Read the model definition and answer for the solid it produces. Units are mm, in the model's axes. Face numbers are marked on the shaded views. A direction names the side the tool comes from. Coordinates: 2 decimals unless noted, no trailing zeros. Loops run counter-clockwise (first coordinate to the right, second up) from the corner with the lowest first, then second, coordinate; pieces in that order, holes last.
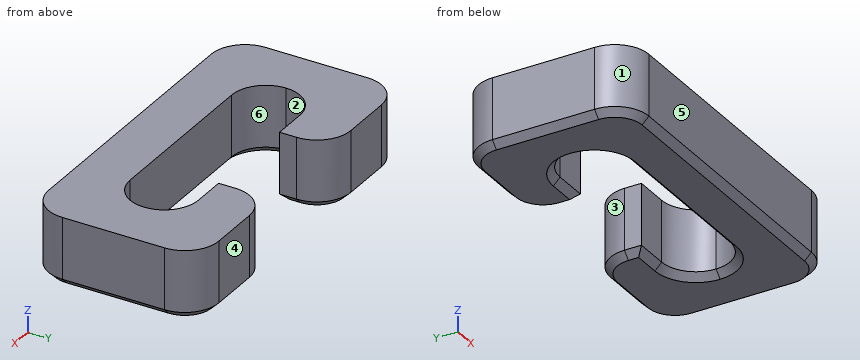
from build123d import *

# Parameters (mm, degrees)
F1_DEPTH = 2
F2_R     = 0.99999
F3_SIZE  = 0.2


# Not quite as in the source:
# - a fillet or chamfer is up to 0.001 mm smaller than in the source, because OpenCascade refuses the exact size


with BuildPart() as f1:
    # F0 (on Top) → F1 (new body)
    with BuildSketch(Plane.XY):
        Polygon((3.5, 0), (0, 0), (-3.5, 0), (-3.5, 2), (-1.5, 2), (-1.5, 3.5), (-5, 3.5), (-5, -1.5), (0, -1.5), (5, -1.5), (5, 3.5), (1.5, 3.5), (1.5, 2), (3.5, 2), align=None)
    extrude(amount=F1_DEPTH)

    # F2 (radius 1 in the source; OpenCascade refuses exactly that, so slightly less here)
    f2_edges = [f1.edges().sort_by_distance(p)[0] for p in [
        (-1.5, 3.5, 1),
        (1.5, 3.5, 1),
        (5, 3.5, 1),
        (5, -1.5, 1),
        (-5, -1.5, 1),
        (-5, 3.5, 1),
        (-3.5, 2, 1),
        (-3.5, 0, 1),
        (3.5, 2, 1),
        (3.5, 0, 1),
    ]]
    fillet(f2_edges, radius=F2_R)

    # F3
    f3_edges = [f1.edges().sort_by_distance(p)[0] for p in [
        (0, 0, 0),
        (3.20711, 0.29289, 0),
        (-3.20711, 0.29289, 0),
        (3.5, 1, 0),
        (-3.5, 1, 0),
        (3.20711, 1.70711, 0),
        (-3.20711, 1.70711, 0),
        (2.000005, 2, 0),
        (-2.000005, 2, 0),
        (1.5, 2.250005, 0),
        (-1.5, 2.250005, 0),
        (1.79289, 3.20711, 0),
        (-1.79289, 3.20711, 0),
        (3.25, 3.5, 0),
        (-3.25, 3.5, 0),
        (4.70711, 3.20711, 0),
        (-4.70711, 3.20711, 0),
        (5, 1, 0),
        (-5, 1, 0),
        (4.70711, -1.20711, 0),
        (-4.70711, -1.20711, 0),
        (0, -1.5, 0),
    ]]
    chamfer(f3_edges, length=F3_SIZE)


solid = f1.part
Item 1: A cutting plane is placed at B-B on x = 0.5. Determine the outline of the cut face in (y, z).
Numbers:
outline: (-1.5, 0.2) - (-1.3, 0) - (-0.2, 0) - (0, 0.2) - (0, 2) - (-1.5, 2) - close
Item 2: Which of the six approach directions +Z, -Z, +X, -X, +Y, -Y give full straight-line access (tool end or side, diameter ignored) to the marked faces 1, 2 and 3?
Numbers:
face 1: +Z, -Z, -X, -Y
face 2: +Z, -Z
face 3: +Z, -Z, +Y
Item 3: Determine the mould class of the marked faces 4, 5 and 6 for opening direction Y: released by +Y, released by -Y, zero draft, split by the parting line, or undercut.
Numbers:
face 4: released by +Y
face 5: released by -Y
face 6: undercut
Item 4: Find the intervals of material crossed by line 1 along X through (y, z) = (2.5, 1.4); line 2 along Y through (x, z) = (-2.5, 1.75); line 3 along Y through (x, z) = (-2, 0.5), in increasing order.
Numbers:
line 1: x = -5 to -1.5, 1.5 to 5
line 2: y = -1.5 to 0, 2 to 3.5
line 3: y = -1.5 to 0, 2 to 3.37
